For this review, use the dimensioned drawing (mm, ordinates from the lowest corner) and the shaded views. Coordinates: 2 decimals unless noted, no trailing zeros. Write each loop counter-clockwise with the first axis right and the second up, starting at its lowest first coordinate (ties: lowest second). Pieces come first, ordered by that corner, then holes. Notation, with made-up numbers: M -34,47 L 12,47 A10 ccw 12,66 Z; hole C -5,-28.75 d6. An arc over 180 degrees is marked long. Return JSON: item names as keys, results as strings.
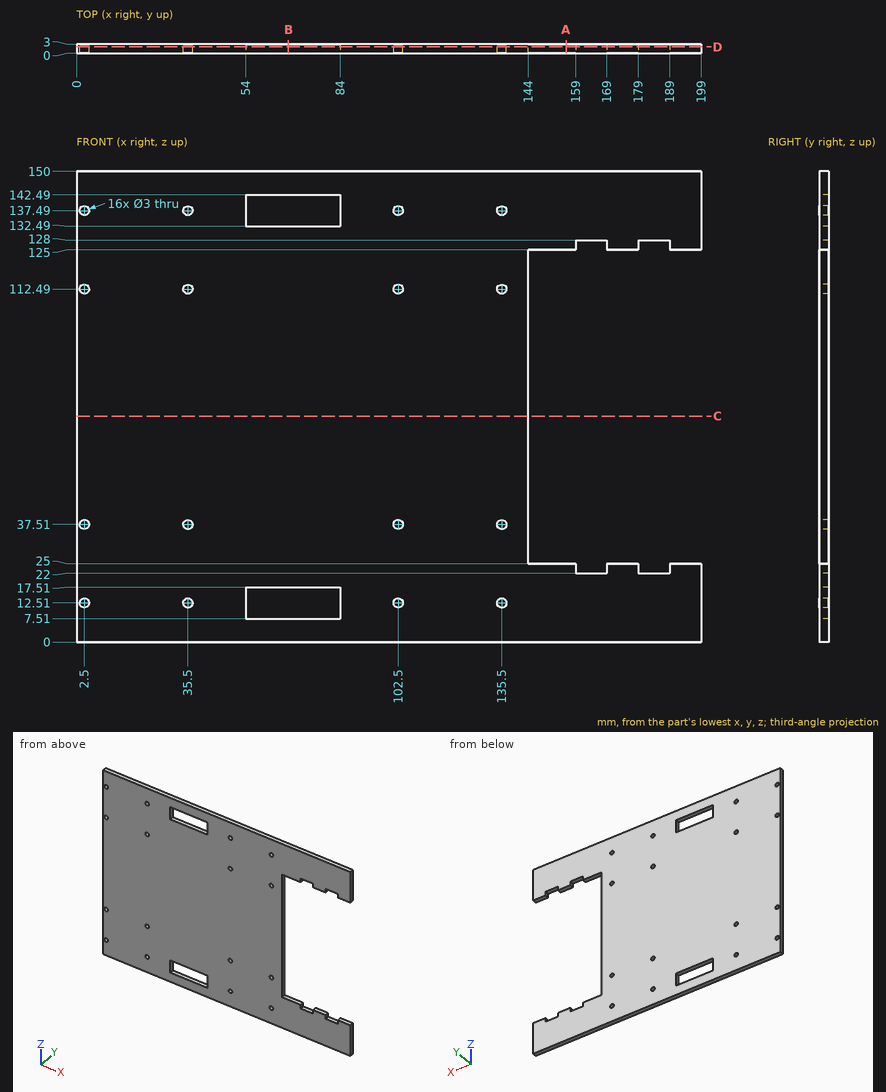
1. Clearance check with a flat-ended pin moving along its axis: pin 1 Ø2.5 at (x, z) = (35.5, 112.49) entering from -Y. State where the tip first meets the part, or that it passes through.
Checks:
{"pin 1": "through"}
2. We need section A-A (x = 156). State the section outline as (y, z) points.
Checks:
{"outline": "M 0,0 L 3,0 L 3,25 L 0,25 Z; M 0,125 L 3,125 L 3,150 L 0,150 Z"}
3. Wall thickness on L1, parallel to X at y = 1.55, z = 112.49; L2, parallel to Z at x = 59, y = 0.4; L3, parallel to X at y = 1.2, z = 24.5: over which ranges is each line inside the solid? List them lowest first. Write a range as from..to.
Checks:
{"L1": "0..1, 4..34, 37..101, 104..134, 137..144", "L2": "0..7.51, 17.51..132.49, 142.49..150", "L3": "0..159, 169..179, 189..199"}
4. We need section D-D (y = 2.1). Give the number of separate pieces and of enclosed holes in the cut face, plus the area to 3 significant figures.
Checks:
{"separate pieces": "1", "enclosed holes": "18", "area": "23,500 mm2"}
5. We need section B-B (x = 67.5). State the section outline as (y, z) points, plus the area to 3 significant figures.
Checks:
{"outline": "M 0,0 L 3,0 L 3,7.51 L 0,7.51 Z; M 0,17.51 L 3,17.51 L 3,132.49 L 0,132.49 Z; M 0,142.49 L 3,142.49 L 3,150 L 0,150 Z", "area": "390 mm2"}
6. We need section C-C (z = 72). State the section outline as (x, y) points, plus the area to 3 significant figures.
Checks:
{"outline": "M 0,0 L 144,0 L 144,3 L 0,3 Z", "area": "432 mm2"}
